Model file for the job. Use its own axes, mm. Face numbers are marked on the shaded views. Coordinates: 2 decimals unless noted, no trailing zeros. Loops run counter-clockwise (first coordinate to the right, second up) from the corner with the lowest first, then second, coordinate; pieces in that order, holes last.
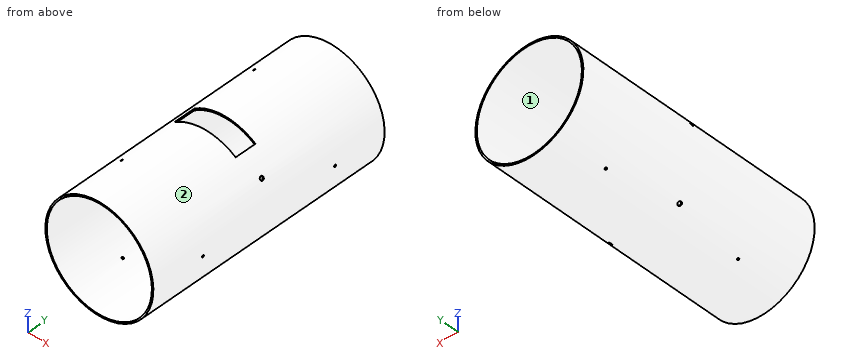
from build123d import *

# Parameters (mm, degrees)
SKETCH1_R               = 76.2
SKETCH1_R_2             = 74.168
BOSS_EXTRUDE1_DEPTH     = 355.6
SKETCH2_W               = 86.36
SKETCH2_H               = 30.48
CUT_EXTRUDE1_DEPTH      = 90.424
SKETCH3_R               = 2.7305
CUT_EXTRUDE2_DEPTH      = 2.54
CIRPATTERN1_COUNT       = 4
CIRPATTERN1_ANGLE       = 240
CUT_EXTRUDE3_REACH      = 378.288
CUT_EXTRUDE3_END_RADIUS = 76.2
SKETCH4_R               = 1.41224
CIRPATTERN2_COUNT       = 3


with BuildPart() as part:
    # Sketch1 → Boss-Extrude1 (new body)
    with BuildSketch(Plane(origin=(0, 0, 0), x_dir=(1, 0, 0), z_dir=(0, 1, 0))):
        with Locations(Location((0, 0, 0), (0, 0, 270))):
            Circle(SKETCH1_R)
        with Locations(Location((0, 0, 0), (0, 0, 270))):
            Circle(SKETCH1_R_2, mode=Mode.SUBTRACT)
    extrude(amount=BOSS_EXTRUDE1_DEPTH)

    # Sketch2 → Cut-Extrude1 (cut)
    with BuildSketch(Plane.XY):
        with Locations((0, 177.8)):
            Rectangle(SKETCH2_W, SKETCH2_H)
    extrude(amount=CUT_EXTRUDE1_DEPTH, mode=Mode.SUBTRACT)

    # Sketch3 → Cut-Extrude2 (cut)
    with BuildSketch(Plane(origin=(-65.991135768, 0, 38.1), x_dir=(0, -1, 0), z_dir=(-0.8660254037844416, 0, 0.49999999999999495))):
        with Locations(Location((-177.8, 0, 0), (0, 0, 90))):
            Circle(SKETCH3_R)
    cut_extrude2 = extrude(amount=-CUT_EXTRUDE2_DEPTH, mode=Mode.SUBTRACT)

    # CirPattern1: Cut-Extrude2 ×4 about axis
    cirpattern1_axis = Axis((0, 355.6, 0), (0, -1, 0))
    for i in range(1, CIRPATTERN1_COUNT):
        add(cut_extrude2.rotate(cirpattern1_axis, i * CIRPATTERN1_ANGLE / (CIRPATTERN1_COUNT - 1)), mode=Mode.SUBTRACT)

    # Cut-Extrude3: up to this cylinder (the profile starts inside it)
    cut_extrude3_end = Plane(origin=(0, 177.8, 0), z_dir=(0, -1, 0)) * Cylinder(CUT_EXTRUDE3_END_RADIUS, 1113.176, mode=Mode.PRIVATE)
    # Sketch4 → Cut-Extrude3 (cut, up to the surface)
    with BuildSketch(Plane(origin=(0, 0, 20.417728463), x_dir=(0, -1, 0), z_dir=(-1, 0, 0)), mode=Mode.PRIVATE) as cut_extrude3_sk1:
        with Locations(Location((-76.2, -20.417728463, 0), (0, 0, 90))):
            Circle(SKETCH4_R)
    cut_extrude3_tool1 = extrude(cut_extrude3_sk1.sketch, amount=-CUT_EXTRUDE3_REACH, mode=Mode.PRIVATE) & cut_extrude3_end
    # Sketch4 → Cut-Extrude3 (cut, up to the surface)
    with BuildSketch(Plane(origin=(0, 0, 20.417728463), x_dir=(0, -1, 0), z_dir=(-1, 0, 0)), mode=Mode.PRIVATE) as cut_extrude3_sk2:
        with Locations(Location((-279.4, -20.417728463, 0), (0, 0, 90))):
            Circle(SKETCH4_R)
    cut_extrude3_tool2 = extrude(cut_extrude3_sk2.sketch, amount=-CUT_EXTRUDE3_REACH, mode=Mode.PRIVATE) & cut_extrude3_end
    cut_extrude3 = cut_extrude3_tool1.solids().sort_by_distance((0, 76.2, 0))[0] + cut_extrude3_tool2.solids().sort_by_distance((0, 279.4, 0))[0]
    add(cut_extrude3, mode=Mode.SUBTRACT)

    # CirPattern2: Cut-Extrude3 ×3 about axis
    cirpattern2_axis = Axis((0, 355.6, 0), (0, 1, 0))
    for i in range(1, CIRPATTERN2_COUNT):
        add(cut_extrude3.rotate(cirpattern2_axis, i * 360 / CIRPATTERN2_COUNT), mode=Mode.SUBTRACT)


solid = part.part
Q1. Slice it at D-D (x = -55). List the corners of the cut face in (y, z), and give its area (3 significant figures).
Answers:
outline: (0, -52.74) - (355.6, -52.74) - (355.6, -49.76) - (0, -49.76) - close; (0, 49.76) - (355.6, 49.76) - (355.6, 52.74) - (0, 52.74) - close
area: 2,120 mm2
Q2. Mould opens along X. For the marked faces 1 and 2 say: +X half, -X half, draft (parallel to the pull), parting line (faces both ways), or undercut.
Answers:
face 1: undercut
face 2: parting line
Q3. Drill centre lines: line 1 (Y direction, x = 75.6, z = 0); line 2 (X direction, y = 170, z = 0); line 3 (X direction, y = 106, z = 7). Where is each one in solid material? Low to high.
Answers:
line 1: y = 0 to 74.79, 77.61 to 277.99, 280.81 to 355.6
line 2: x = -76.2 to -74.17, 74.17 to 76.2
line 3: x = -75.88 to -73.84, 73.84 to 75.88
Q4. Slice it at A-A (x = -22). List the corners of the cut face in (y, z), and give its area (3 significant figures).
Answers:
outline: (0, -72.96) - (355.6, -72.96) - (355.6, -70.83) - (0, -70.83) - close; (0, 70.83) - (162.56, 70.83) - (162.56, 72.96) - (0, 72.96) - close; (193.04, 70.83) - (355.6, 70.83) - (355.6, 72.96) - (193.04, 72.96) - close
area: 1,450 mm2
Q5. Flat gauge pins, fed straight in: P1, Ø8, axis at y = 206, z = -5.5, coming from the +X side; P2, Ø2, axis at y = 183, z = 61.5, coming from the +X side; P3, Ø12, axis at y = 153, z = -22.5, coming from the +X side; P4, Ø5, axis at x = -11.5, z = 68.5, coming from the +Y side. Where does each tip first touch, or does it go through?
Answers:
P1: stops at x = 76.19
P2: stops at x = 46.33
P3: stops at x = 74.39
P4: passes through
Q6. Slice it at C-C (y = 133.5). List the corners of the cut face in (x, z).
Answers:
outline: circle Ø152.4 at (0, 0); hole circle Ø148.34 at (0, 0)
Q7. Slice it at B-B (z = -46). List the corners of the cut face in (x, y), and give its area (3 significant figures).
Answers:
outline: (-60.75, 0) - (-58.18, 0) - (-58.18, 355.6) - (-60.75, 355.6) - close; (58.18, 0) - (60.75, 0) - (60.75, 355.6) - (58.18, 355.6) - close
area: 1,830 mm2
